CAD build for the part. Positions are in the model's coordinates, mm. A direction names the side the tool comes from. Coordinates: 2 decimals unless noted, no trailing zeros. Loops run counter-clockwise (first coordinate to the right, second up) from the corner with the lowest first, then second, coordinate; pieces in that order, holes last. Notation, with made-up numbers: (60, 4) -> (106, 4) arc R27 ccw to (106, 43) -> close; hole circle Ø7 at (34, 11). An arc over 180 degrees is marked (long way). Write item = value, one per line. Start each with the question number.
(1) Flat gauge pins, fed straight in: P1, Ø0.6, axis at y = 91, z = 1, coming from the +X side; P2, Ø0.6, axis at y = 91.5, z = 0.5, coming from the -X side; P3, Ø0.6, axis at y = 134, z = 0.5, coming from the +X side. Where does each tip first touch, or does it go through?
(2) Tool access for faces 1 (the face through (-36, 137.582, 1)), 2 (the face through (11.997, 81.298, 0.986)), 3 (the face through (-1, 105, 0)), 4 (the face through (8.45, 94.21, 0.99)): list every direction of +Z, -Z, +X, -X, +Y, -Y with a clear straight run to the whole face (end or side of a thin tool).
(3) Band-saw the part on A-A (x = 3.5). Write the cut outline in (y, z).
(4) Band-saw the part on C-C (z = 0.3). Count the separate pieces of the cut face and the enclosed holes in it, and give its area (3 significant figures).
(5) Drill centre lines: line 1 (Y direction, x = -17.25, z = 1); line 2 (Y direction, x = -2, z = 1.9); line 3 (X direction, y = 119, z = 0.8). Where is each one in solid material? Low to high. Write a range as from..to.
(6) Band-saw the part on B-B (x = -34.05). Write the cut outline in (y, z).
(7) Band-saw the part on D-D (x = 23.5). Write the cut outline in (y, z), and give its area (3 significant figures).
(8) Pull direction Y, two halves, no side cores. Call faces 5 (the face through (-30.052, 89, 1)), 6 (the face through (24.8, 83.24, 0.99)), 7 (the face through (-32.5, 114, 1)): +Y half, -Y half, draft (parallel to the pull), parting line (faces both ways), or undercut.
```python
from build123d import *

# Parameters (mm, degrees)
SKETCH_1_R      = 2.75
EXTRUDE_1_DEPTH = 2


with BuildPart() as part:
    # 草图1 → 凸台-拉伸1 (new body)
    with BuildSketch(Plane.XY):
        with BuildLine():
            Line((-24.447800114, 142.867788384), (-29.015821613, 138.834288737))
            ThreePointArc((-29.015821613, 138.834288737), (-30.556091587, 137.905760103), (-32.325263946, 137.582300402))
            Line((-32.325263946, 137.582300402), (-39.033457742, 137.582300402))
            ThreePointArc((-39.033457742, 137.582300402), (-40.802630101, 137.2588407), (-42.342900075, 136.330312067))
            Line((-42.342900075, 136.330312067), (-44.480254451, 134.443057788))
            ThreePointArc((-44.480254451, 134.443057788), (-45.728619247, 132.750865708), (-46.170812117, 130.695046123))
            Line((-46.170812117, 130.695046123), (-46.170812117, 101.166813467))
            ThreePointArc((-46.170812117, 101.166813467), (-45.154526002, 98.050429516), (-42.496431366, 96.132300402))
            Line((-42.496431366, 96.132300402), (-35.6, 93.92431119))
            Line((-35.6, 93.92431119), (-30.05244945, 90.888042458))
            Line((-30.05244945, 90.888042458), (-30.05244945, 87.84217512))
            Line((-30.05244945, 87.84217512), (-19.688242157, 78.763336754))
            Line((-19.688242157, 78.763336754), (-14.532154357, 78.763336754))
            Line((-14.532154357, 78.763336754), (-9.532154357, 83.763336754))
            Line((-9.532154357, 83.763336754), (9.532154357, 83.763336754))
            Line((9.532154357, 83.763336754), (14.532154357, 78.763336754))
            Line((14.532154357, 78.763336754), (19.688242157, 78.763336754))
            Line((19.688242157, 78.763336754), (30.05244945, 87.84217512))
            Line((30.05244945, 87.84217512), (30.05244945, 90.888042458))
            Line((30.05244945, 90.888042458), (35.6, 93.92431119))
            Line((35.6, 93.92431119), (42.496431366, 96.132300402))
            ThreePointArc((42.496431366, 96.132300402), (45.154526002, 98.050429516), (46.170812117, 101.166813467))
            Line((46.170812117, 101.166813467), (46.170812117, 130.695046123))
            ThreePointArc((46.170812117, 130.695046123), (45.728619247, 132.750865708), (44.480254451, 134.443057788))
            Line((44.480254451, 134.443057788), (42.342900075, 136.330312067))
            ThreePointArc((42.342900075, 136.330312067), (40.802630101, 137.2588407), (39.033457742, 137.582300402))
            Line((39.033457742, 137.582300402), (32.472417217, 137.582300402))
            ThreePointArc((32.472417217, 137.582300402), (30.584617738, 137.952374579), (28.976268595, 139.007815151))
            Line((28.976268595, 139.007815151), (25.245537252, 142.656785653))
            ThreePointArc((25.245537252, 142.656785653), (23.637188108, 143.712226225), (21.74938863, 144.082300402))
            Line((21.74938863, 144.082300402), (15.032154357, 144.082300402))
            Line((15.032154357, 144.082300402), (9.532154357, 138.582300402))
            Line((9.532154357, 138.582300402), (-9.532154357, 138.582300402))
            Line((-9.532154357, 138.582300402), (-15.032154357, 144.082300402))
            Line((-15.032154357, 144.082300402), (-21.74938863, 144.082300402))
            ThreePointArc((-21.74938863, 144.082300402), (-23.190499918, 143.679240794), (-24.447800114, 142.867788384))
        make_face()
        with Locations((39.335406059, 129.082300402)):
            Circle(SKETCH_1_R, mode=Mode.SUBTRACT)
        with Locations((39.335406059, 104.082300402)):
            Circle(SKETCH_1_R, mode=Mode.SUBTRACT)
        with Locations((17.23796389, 84.763336754)):
            Circle(SKETCH_1_R, mode=Mode.SUBTRACT)
        with Locations(Location((-17.23796389, 84.763336754, 0), (0, 0, 180))):
            Circle(SKETCH_1_R, mode=Mode.SUBTRACT)
        with Locations(Location((-39.335406059, 104.082300402, 0), (0, 0, 180))):
            Circle(SKETCH_1_R, mode=Mode.SUBTRACT)
        with Locations(Location((-39.335406059, 129.082300402, 0), (0, 0, 180))):
            Circle(SKETCH_1_R, mode=Mode.SUBTRACT)
        with Locations((17.25, 134.317818161)):
            Circle(SKETCH_1_R, mode=Mode.SUBTRACT)
        with Locations(Location((17.25, 99.817818161, 0), (0, 0, 180))):
            Circle(SKETCH_1_R, mode=Mode.SUBTRACT)
        with Locations((-17.25, 99.817818161)):
            Circle(SKETCH_1_R, mode=Mode.SUBTRACT)
        with Locations(Location((-17.25, 134.317818161, 0), (0, 0, 180))):
            Circle(SKETCH_1_R, mode=Mode.SUBTRACT)
        Polygon((7.105388598, 96.132300402), (-7.105388598, 96.132300402), (-9.761471208, 92.339021317), (-9.761471208, 90.339021317), (9.761471208, 90.339021317), (9.761471208, 92.339021317), align=None, mode=Mode.SUBTRACT)
        with BuildLine():
            Line((-35.6, 116.582300402), (-35.6, 112.082300402))
            ThreePointArc((-35.6, 112.082300402), (-34.05, 110.532300402), (-32.5, 112.082300402))
            Line((-32.5, 112.082300402), (-32.5, 116.582300402))
            ThreePointArc((-32.5, 116.582300402), (-34.05, 118.132300402), (-35.6, 116.582300402))
        make_face(mode=Mode.SUBTRACT)
        with BuildLine():
            Line((35.6, 116.582300402), (35.6, 112.082300402))
            ThreePointArc((35.6, 112.082300402), (34.05, 110.532300402), (32.5, 112.082300402))
            Line((32.5, 112.082300402), (32.5, 116.582300402))
            ThreePointArc((32.5, 116.582300402), (34.05, 118.132300402), (35.6, 116.582300402))
        make_face(mode=Mode.SUBTRACT)
        Polygon((-17.12762315, 113.853040841), (-11.506056087, 107.618637195), (11.506056087, 107.618637195), (17.12762315, 113.853040841), (17.12762315, 120.282595482), (11.506056087, 126.516999128), (-11.506056087, 126.516999128), (-17.12762315, 120.282595482), align=None, mode=Mode.SUBTRACT)
        Polygon((-7.105388598, 129.79821171), (7.105388598, 129.79821171), (9.761471208, 133.591490795), (9.761471208, 135.591490795), (-9.761471208, 135.591490795), (-9.761471208, 133.591490795), align=None, mode=Mode.SUBTRACT)
        with BuildLine():
            Line((-22.20520244, 127.943672987), (-22.20520244, 106.191963336))
            ThreePointArc((-22.20520244, 106.191963336), (-24.592663446, 103.80450233), (-26.980124451, 106.191963336))
            Line((-26.980124451, 106.191963336), (-26.980124451, 127.943672987))
            ThreePointArc((-26.980124451, 127.943672987), (-24.592663446, 130.331133992), (-22.20520244, 127.943672987))
        make_face(mode=Mode.SUBTRACT)
        with BuildLine():
            Line((22.20520244, 127.943672987), (22.20520244, 106.191963336))
            ThreePointArc((22.20520244, 106.191963336), (24.592663446, 103.80450233), (26.980124451, 106.191963336))
            Line((26.980124451, 106.191963336), (26.980124451, 127.943672987))
            ThreePointArc((26.980124451, 127.943672987), (24.592663446, 130.331133992), (22.20520244, 127.943672987))
        make_face(mode=Mode.SUBTRACT)
    extrude(amount=EXTRUDE_1_DEPTH)


solid = part.part
```
Findings below:
q1.P1 = 30.81
q1.P2 = -31.72
q1.P3 = 45.17
q2.face_1 = +Z, -Z, -X, +Y
q2.face_2 = +Z, -Z, -Y
q2.face_3 = -Z, +X, -X, +Y, -Y
q2.face_4 = +Z, -Z
q3.outline = (83.76, 0) -> (90.34, 0) -> (90.34, 2) -> (83.76, 2) -> close; (96.13, 0) -> (107.62, 0) -> (107.62, 2) -> (96.13, 2) -> close; (126.52, 0) -> (129.8, 0) -> (129.8, 2) -> (126.52, 2) -> close; (135.59, 0) -> (138.58, 0) -> (138.58, 2) -> (135.59, 2) -> close
q4.separate_pieces = 1
q4.enclosed_holes = 17
q4.area = 3,580 mm²
q5.line_1 = 78.76..82.01, 87.51..97.07, 102.57..131.57, 137.07..144.08
q5.line_2 = 83.76..90.34, 96.13..107.62, 126.52..129.8, 135.59..138.58
q5.line_3 = -46.17..-26.98, -22.21..-17.13, 17.13..22.21, 26.98..46.17
q6.outline = (93.08, 0) -> (110.53, 0) -> (110.53, 2) -> (93.08, 2) -> close; (118.13, 0) -> (137.58, 0) -> (137.58, 2) -> (118.13, 2) -> close
q7.outline = (82.1, 0) -> (104.07, 0) -> (104.07, 2) -> (82.1, 2) -> close; (130.07, 0) -> (143.77, 0) -> (143.77, 2) -> (130.07, 2) -> close
q7.area = 71.3 mm²
q8.face_5 = draft
q8.face_6 = -Y half
q8.face_7 = undercut
